The drawing under review shows one solid part. Ordinate dimensions are in mm from its lowest x, y, z. Round coordinates to 2 decimals unless told otherwise and drop trailing zeros. Order: outer loops, then holes, each group sorted by start corner. A loop starts at its lowest first (then second) coordinate and runs counter-clockwise, first axis right, second up. Notation, with made-up numbers: (84, 17) -> (116, 17) arc R6 cw to (116, 25) -> close; hole circle Ø10 at (7, -2.75). An arc over 180 degrees is marked (long way). Put each result on its own line as item: value. Start each with the question number.
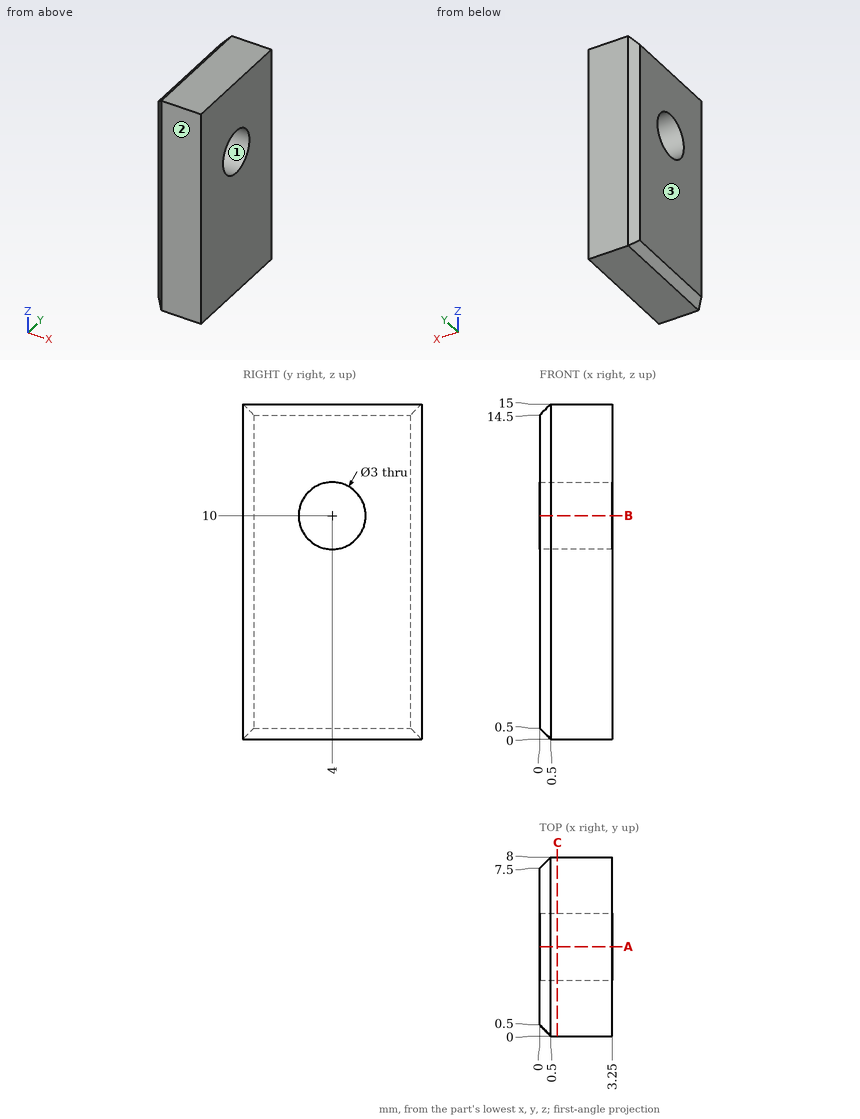
Item 1: Consider section A-A, the plane y = 4. Write out the cut boundary in (x, z), plus the area to 4 significant figures.
Item 2: Consider section C-C, the plane x = 0.8. Write out the cut boundary in (y, z).
Item 3: Consider section B-B, the plane z = 10. Write out the cut boundary in (x, y), plus the area to 3 significant figures.
Item 4: For L1, parallel to Y at x = 2.35, z = 10; L2, parallel to Z at x = 0.8, y = 5; L3, parallel to Z at x = 1.95, y = 3.25, list the stretches that pass through material, from the lowest coordinate up.
Item 5: Insertion check: pin 1 Ø3.5 at (y, z) = (4, 10) entering from -X. The pin has a flat end and moves straight along its axis. Give the tip position at first contact, or say it passes through.
Item 6: Mouldability with a two-part tool opening along Y and no side actions: class the marked faces 1, 2 and 3 as +Y half, -Y half, draft (parallel to the pull), parting line (faces both ways), or undercut.
Evaluation:
1. outline: (0, 0.5) -> (0.5, 0) -> (3.25, 0) -> (3.25, 8.5) -> (0, 8.5) -> close; (0, 11.5) -> (3.25, 11.5) -> (3.25, 15) -> (0.5, 15) -> (0, 14.5) -> close
1. area: 38.75 mm^2
2. outline: (0, 0) -> (8, 0) -> (8, 15) -> (0, 15) -> close; hole circle Ø3 at (4, 10)
3. outline: (0, 0.5) -> (0.5, 0) -> (3.25, 0) -> (3.25, 2.5) -> (0, 2.5) -> close; (0, 5.5) -> (3.25, 5.5) -> (3.25, 8) -> (0.5, 8) -> (0, 7.5) -> close
3. area: 16.0 mm^2
4. L1: y = 0 to 2.5, 5.5 to 8
4. L2: z = 0 to 8.88, 11.12 to 15
4. L3: z = 0 to 8.7, 11.3 to 15
5. pin 1: stops at x = 0
6. face 1: undercut
6. face 2: -Y half
6. face 3: draft
